from build123d import *

# Parameters (mm, degrees)
F0_W     = 30.67
F0_H     = 30.67
F1_DEPTH = 1
F0_W_2   = 12.1056904889
F0_H_2   = 1.4927708568
F0_W_3   = 1.4087211761
F0_H_3   = 4.1082873123
F2_DEPTH = 1.8


# Not quite as in the source:
# - a feature names something its author has since deleted; it is built from what else it names


with BuildPart() as f1:
    # F0 (on Top) → F1 (new body)
    with BuildSketch(Plane.XY):
        Rectangle(F0_W, F0_H)
        with BuildLine():
            ThreePointArc((-8.8560749891, 11.0999971075), (6.1596970362, 12.7944570976), (14.2, 0))
            ThreePointArc((14.2, 0), (2.9118804142, -13.8982355878), (-13.0057679512, -5.7))
            Line((-13.0057679512, -5.7), (-14.0999610525, -5.7))
            Line((-14.0999610525, -5.7), (-14.0999610525, -1.6825867938))
            ThreePointArc((-14.0999610525, -1.6825867938), (-14.2, 0), (-14.0999610525, 1.6825867938))
            Line((-14.0999610525, 1.6825867938), (-14.0999610525, 5.7))
            Line((-14.0999610525, 5.7), (-14.0999610525, 11.0999971075))
            Line((-14.0999610525, 11.0999971075), (-8.8560749891, 11.0999971075))
        make_face(mode=Mode.SUBTRACT)
        with BuildLine():
            ThreePointArc((-14.0999610525, 1.6825867938), (-14.2, 0), (-14.0999610525, -1.6825867938))
            Line((-14.0999610525, -1.6825867938), (-14.0999610525, 1.6825867938))
        make_face()
    extrude(amount=-F1_DEPTH)



with BuildPart() as f1b:
    # F0 (on Top) → F1, piece 2 (new body)
    with BuildSketch(Plane.XY):
        with BuildLine():
            Line((2.9913177714, -5.7), (-9.1143727175, -5.7))
            ThreePointArc((-9.1143727175, -5.7), (-3.1266086976, -10.2852600601), (4.4000389475, -9.8082873123))
            ThreePointArc((4.4000389475, -9.8082873123), (10.7500389475, 0), (4.4000389475, 9.8082873123))
            Line((4.4000389475, 9.8082873123), (4.4000389475, 5.7))
            Line((4.4000389475, 5.7), (4.4000389475, 4.2072320357))
            Line((4.4000389475, 4.2072320357), (4.4000389475, -4.2072320357))
            Line((4.4000389475, -4.2072320357), (4.4000389475, -5.7))
            Line((4.4000389475, -5.7), (2.9913177714, -5.7))
        make_face()
        Polygon((2.9913177714, -4.2072291432), (2.9913177714, -5.7), (4.4000389475, -5.7), (4.4000389475, -4.2072320357), (4.4000389475, 4.2072320357), (4.4000389475, 5.7), (2.9913177714, 5.7), (2.9913177714, 4.2072291432), align=None)
        with Locations((-3.0615274731, -4.9536145716)):
            Rectangle(F0_W_2, F0_H_2)
        Polygon((2.9913177714, -4.2072291432), (2.9913177714, -5.7), (4.4000389475, -5.7), (4.4000389475, -4.2072320357), (4.4000389475, 4.2072320357), (4.4000389475, 5.7), (2.9913177714, 5.7), (2.9913177714, 4.2072291432), align=None)
        with Locations((3.6956783594, 7.7541436561)):
            Rectangle(F0_W_3, F0_H_3)
    extrude(amount=-F1_DEPTH)


with BuildPart() as f1_1:
    add(f1.part)

    add(f1b.part)  # F2 merges F1b
    # F0 (on Top) → F2 (join)
    with BuildSketch(Plane.XY):
        Rectangle(F0_W, F0_H)
        with BuildLine():
            ThreePointArc((-8.8560749891, 11.0999971075), (6.1596970362, 12.7944570976), (14.2, 0))
            ThreePointArc((14.2, 0), (2.9118804142, -13.8982355878), (-13.0057679512, -5.7))
            Line((-13.0057679512, -5.7), (-14.0999610525, -5.7))
            Line((-14.0999610525, -5.7), (-14.0999610525, -1.6825867938))
            ThreePointArc((-14.0999610525, -1.6825867938), (-14.2, 0), (-14.0999610525, 1.6825867938))
            Line((-14.0999610525, 1.6825867938), (-14.0999610525, 5.7))
            Line((-14.0999610525, 5.7), (-14.0999610525, 11.0999971075))
            Line((-14.0999610525, 11.0999971075), (-8.8560749891, 11.0999971075))
        make_face(mode=Mode.SUBTRACT)
        with BuildLine():
            ThreePointArc((-13.0057679512, -5.7), (2.9118804142, -13.8982355878), (14.2, 0))
            ThreePointArc((14.2, 0), (6.1596970362, 12.7944570976), (-8.8560749891, 11.0999971075))
            Line((-8.8560749891, 11.0999971075), (2.9913177714, 11.0999971075))
            Line((2.9913177714, 11.0999971075), (4.4000389475, 11.0999971075))
            Line((4.4000389475, 11.0999971075), (4.4000389475, 9.8082873123))
            ThreePointArc((4.4000389475, 9.8082873123), (10.7500389475, 0), (4.4000389475, -9.8082873123))
            ThreePointArc((4.4000389475, -9.8082873123), (-3.1266086976, -10.2852600601), (-9.1143727175, -5.7))
            Line((-9.1143727175, -5.7), (-13.0057679512, -5.7))
        make_face()
        with BuildLine():
            Line((2.9913177714, -5.7), (-9.1143727175, -5.7))
            ThreePointArc((-9.1143727175, -5.7), (-3.1266086976, -10.2852600601), (4.4000389475, -9.8082873123))
            ThreePointArc((4.4000389475, -9.8082873123), (10.7500389475, 0), (4.4000389475, 9.8082873123))
            Line((4.4000389475, 9.8082873123), (4.4000389475, 5.7))
            Line((4.4000389475, 5.7), (4.4000389475, 4.2072320357))
            Line((4.4000389475, 4.2072320357), (4.4000389475, -4.2072320357))
            Line((4.4000389475, -4.2072320357), (4.4000389475, -5.7))
            Line((4.4000389475, -5.7), (2.9913177714, -5.7))
        make_face()
        with BuildLine():
            ThreePointArc((-14.0999610525, 1.6825867938), (-14.2, 0), (-14.0999610525, -1.6825867938))
            Line((-14.0999610525, -1.6825867938), (-14.0999610525, 1.6825867938))
        make_face()
    extrude(amount=F2_DEPTH)


solid = f1_1.part
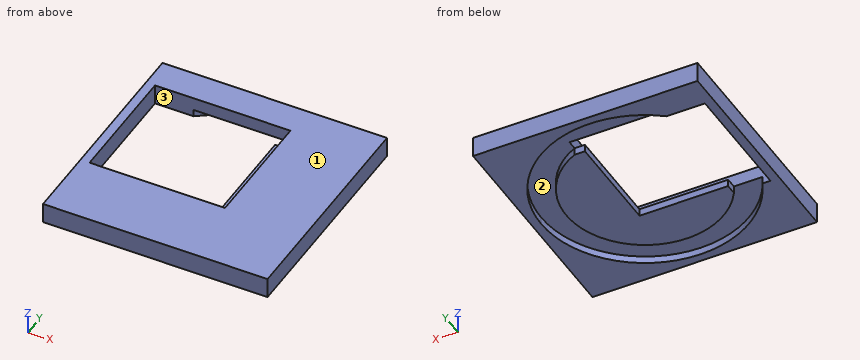
Input: part model. Units: mm. Frame: model coordinates. Face numbers are marked on the shaded views. Round coordinates to 2 decimals unless told otherwise and drop trailing zeros. Loops run counter-clockwise (first coordinate to the right, second up) from the corner with the lowest first, then second, coordinate; pieces in that order, holes last. Notation, with made-up numbers: M 53.25,39 L 112.25,39 A21 ccw 112.25,44 Z; hole C -19.75,-6.75 d6. An arc over 180 degrees is marked long. Answer as CSV lines item,"result". Start each with the question number.
(1) Section C-C, the plane y = 1.5. Output: boundary loops of the cut face in (x, z) (3 decimals), plus the area to 3 significant figures.
(2) Draft query along X for the marked faces 1, 2 and 3. Return one class per face: released by +X, released by -X, zero draft, split by the parting line, or undercut.
(3) Section A-A, the plane x = 0. Output: boundary loops of the cut face in (y, z) (3 decimals), plus the area to 3 significant figures.
(4) Section B-B, the plane z = 1.4. Output: boundary loops of the cut face in (x, y) (3 decimals), plus the area to 3 significant figures.
(5) Section D-D, the plane y = -8.5. Output: boundary loops of the cut face in (x, z) (3 decimals).
(6) Line query: line 1 (X direction, y = 0.5, z = 0.3) (3 decimals); line 2 (Y direction, x = 0, z = 0.35) (3 decimals); line 3 (X direction, y = -9, z = -0.2) (3 decimals). Output: solid intervals per line, ascending. Write a range as [from, to].
Values found:
1,outline,"M -15.335,-1 L -14.1,-1 L -14.1,1.8 L -15.335,1.8 Z; M 2.991,-1 L 10.645,-1 L 10.645,0 L 14.121,0 L 14.121,-1 L 15.335,-1 L 15.335,1.8 L 4.4,1.8 L 4.4,0 L 2.991,0 Z"
1,area,"32.0 mm²"
2,face 1,"zero draft"
2,face 2,"undercut"
2,face 3,"undercut"
3,outline,"M -15.335,-1 L -14.2,-1 L -14.2,0 L -10.75,0 L -10.75,-1 L -4.207,-1 L -4.207,0 L -5.7,0 L -5.7,1.8 L -15.335,1.8 Z; M 11.1,0 L 14.2,0 L 14.2,-1 L 15.335,-1 L 15.335,1.8 L 11.1,1.8 Z"
3,area,"33.8 mm²"
4,outline,"M -15.335,-15.335 L 15.335,-15.335 L 15.335,15.335 L -15.335,15.335 Z; hole M -14.1,-5.7 L 4.4,-5.7 L 4.4,11.1 L -14.1,11.1 Z"
4,area,"630 mm²"
5,outline,"M -15.335,-1 L -11.375,-1 L -11.375,0 L -6.581,0 L -6.581,-1 L 6.581,-1 L 6.581,0 L 11.375,0 L 11.375,-1 L 15.335,-1 L 15.335,1.8 L -15.335,1.8 Z"
6,line 1,"x = [-15.335, -14.1], [4.4, 15.335]"
6,line 2,"y = [-15.335, -5.7], [11.1, 15.335]"
6,line 3,"x = [-15.335, -10.984], [-5.879, 5.879], [10.984, 15.335]"
